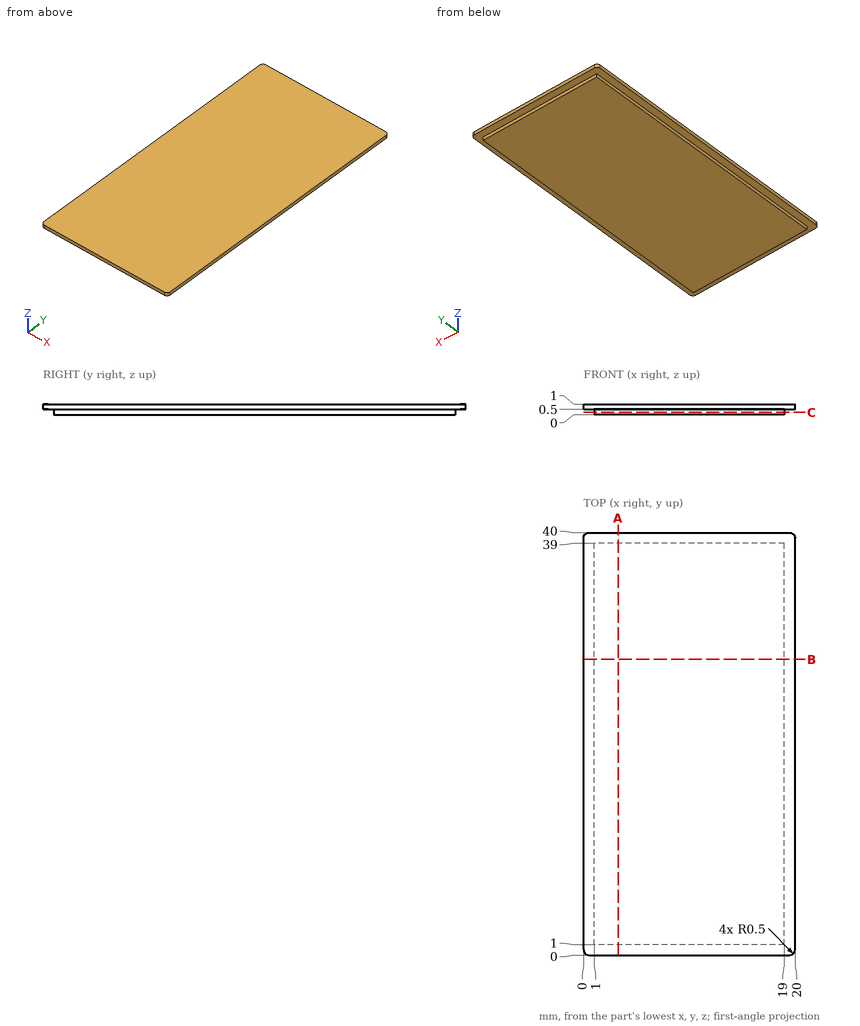
Here's the drawing with two shaded views (mm, measured from the low corner). I have some questions. Coordinates: 2 decimals unless noted, no trailing zeros. Loops run counter-clockwise (first coordinate to the right, second up) from the corner with the lowest first, then second, coordinate; pieces in that order, holes last. Notation, with made-up numbers: M 77,28.25 L 106,28.25 A7 cw 106,37.25 Z; hole C 81,30.5 d7. An arc over 180 degrees is marked long. Return JSON: item names as keys, results as strings. Group by question number.
Item 1: Imagine slicing it at A-A (x = 3.25). Please give me the cut outline in (y, z), and give its area (3 significant figures).
Item 2: Imagine slicing it at B-B (y = 28). Please give me the cut outline in (x, z).
Item 3: Imagine slicing it at C-C (z = 0.2). Please give me the cut outline in (x, y), and give its area (3 significant figures).
Item 4: If I drill on L1, parallel to Y at x = 8, z = 0.1; L2, parallel to X at y = 11, z = 0.1, over which ranges is the centre line in solid material (lowest first)? Write a range as from..to.
Verdict:
{
 "1": {"outline": "M 0,0.5 L 1,0.5 L 1,0 L 39,0 L 39,0.5 L 40,0.5 L 40,1 L 0,1 Z", "area": "39.0 mm^2"},
 "2": {"outline": "M 0,0.5 L 1,0.5 L 1,0 L 19,0 L 19,0.5 L 20,0.5 L 20,1 L 0,1 Z"},
 "3": {"outline": "M 1,1 L 19,1 L 19,39 L 1,39 Z", "area": "684 mm^2"},
 "4": {"L1": "y = 1..39", "L2": "x = 1..19"}
}
